Solid Edge part; units mm, degrees
sketch "Sketch1" plane through (0, 0, 0) normal (0, -1, 0) x (1, 0, 0)
  line L0 (30, 0) -> (18.9422, 160.02)
  line L1 (-19.0139, 161.311) -> (-20, 0)
  line L2 (30, 0) -> (-20, 0)
  arc A0 (-19.0139, 161.311) -> (18.9422, 160.02) centre (-0.0578, 160.02) cw
extrude "Protrusion1" add sketch "Sketch1" against normal blind 10
sketch "Sketch2" plane through (0, 0, 0) normal (0, -1, 0) x (1, 0, 0)
  circle A0 centre (0, 160) radius 10
extrude "ExtrudedCutout_1" cut sketch "Sketch2" against normal blind 10
hole "Hole_1" at (-15.5, 0, 5.5) direction (0, 1, 0) diameter 3.2 end through all counterbore diameter 5.8 counterbore depth 3.4
pattern_linear "Pattern1" count 2 spacing 31 along (1, 0, 0) count 2 spacing 31 along (0, 0, 1) of "Hole_1"
hole "Hole_2" at (0, 10, 21) direction (0, -1, 0) diameter 5.5 end through all counterbore diameter 23 counterbore depth 3
sketch "Sketch3" plane through (0, 0, 89.51) normal (0, -1, 0) x (1, 0, 0)
  line L0 (9.2202, -0.4765) -> (6.2316, -0.7379)
  line L1 (6.1009, 0.7564) -> (6.2316, -0.7379)
  line L2 (14.0705, 1.4536) -> (6.1009, 0.7564)
  line L3 (14.2012, -0.0407) -> (14.0705, 1.4536)
  line L4 (9.2202, -0.4765) -> (14.2012, -0.0407)
  line L5 (14.7241, -6.0178) -> (9.7432, -6.4536)
  line L6 (9.7432, -6.4536) -> (9.3074, -1.4727)
  line L7 (14.2883, -1.0369) -> (9.3074, -1.4727)
  line L8 (14.7241, -6.0178) -> (14.2883, -1.0369)
  line L9 (9.8303, -7.4498) -> (14.8113, -7.014)
  line L10 (14.942, -8.5083) -> (14.8113, -7.014)
  line L11 (6.9725, -9.2056) -> (14.942, -8.5083)
  line L12 (6.8417, -7.7113) -> (6.9725, -9.2056)
  line L13 (6.8417, -7.7113) -> (9.8303, -7.4498)
extrude "ExtrudedProtrusion_2" add sketch "Sketch3" along normal blind 8
sketch "Sketch4" plane through (0, 0, 89.51) normal (0, -1, 0) x (1, 0, 0)
  circle A0 centre (15.8473, -0.0407) radius 1
  circle A1 centre (16.3289, -6.7414) radius 1
extrude "ExtrudedCutout_3" cut sketch "Sketch4" against normal blind 10
sketch "Sketch5" plane through (12.0158, -8, 85.7648) normal (0, -1, 0) x (0.9962, 0, 0.0872)
  line L0 (-5.5, 5) -> (-5.5, -5)
  line L1 (-5.5, -5) -> (2.5, -5)
  line L2 (2.5, -5) -> (2.5, 5)
  line L3 (2.5, 5) -> (-5.5, 5)
extrude "ExtrudedProtrusion_3" add sketch "Sketch5" along normal blind 3
sketch "Sketch6" plane through (0, 0, 89.51) normal (0, -1, 0) x (1, 0, 0)
  line L0 (-12.7631, 16.3965) -> (-4.7936, 15.6993)
  line L1 (-4.7936, 15.6993) -> (-4.9243, 14.205)
  line L2 (-4.9243, 14.205) -> (-12.8939, 14.9022)
  line L3 (-12.8939, 14.9022) -> (-12.7631, 16.3965)
  line L4 (-8.4358, 8.4893) -> (-8, 13.4703)
  line L5 (-8, 13.4703) -> (-12.981, 13.906)
  line L6 (-12.981, 13.906) -> (-13.4168, 8.9251)
  line L7 (-13.4168, 8.9251) -> (-8.4358, 8.4893)
  line L8 (-13.5039, 7.9289) -> (-5.5344, 7.2316)
  line L9 (-5.5344, 7.2316) -> (-5.6651, 5.7373)
  line L10 (-5.6651, 5.7373) -> (-13.6347, 6.4346)
  line L11 (-13.6347, 6.4346) -> (-13.5039, 7.9289)
extrude "ExtrudedProtrusion_4" add sketch "Sketch6" along normal blind 8
sketch "Sketch7" plane through (-10.7084, -8, 100.7077) normal (0, -1, 0) x (0.9962, 0, -0.0872)
  line L0 (5.5, 5) -> (5.5, -5)
  line L1 (5.5, -5) -> (-2.5, -5)
  line L2 (-2.5, -5) -> (-2.5, 5)
  line L3 (-2.5, 5) -> (5.5, 5)
extrude "ExtrudedProtrusion_5" add sketch "Sketch7" along normal blind 3
hole "Hole1" at (-14.1769, 0, 104.0133) direction (0, 1, 0) diameter 2 end up to next
hole "Hole2" at (-14.7852, 0, 97.9993) direction (0, 1, 0) diameter 2 end up to next
fillet "Round_1" [suppressed]
fillet "Round_2" radius 1 4 edges at (-8.7783, -11, 105.5579) (-13.1989, -11, 100.9256) (-9.6499, -11, 95.596) (-5.2293, -11, 100.2283)
fillet "Round_3" radius 1 4 edges at (10.0857, -11, 90.615) (6.5367, -11, 85.2854) (10.9572, -11, 80.653) (14.5062, -11, 85.9826)
fillet "Round_4" [suppressed]
Part model, mm, in its own coordinate system. A direction names the side the tool comes from. Coordinates: 2 decimals unless noted, no trailing zeros. Loops run counter-clockwise (first coordinate to the right, second up) from the corner with the lowest first, then second, coordinate; pieces in that order, holes last. Notation, with made-up numbers: M 30,37 L 80,37 A18 cw 80,67 Z; hole C 19.5,81.5 d5. An arc over 180 degrees is marked long. Use a Markdown table: item, result. Add a question column.
Q1. Cut at A-A (z = 36.5). Write the cut outline in (x, y).
Q2. Probe L1, parallel to Z at x = 0, y = 4; L2, parallel to Z at x = 0, y = 8; L3, parallel to Z at x = -15.5, y = 1.1. List the from-to ranges inside material, lowest first.
Q3. Which spindle directions (+Z, -Z, +X, -X, +Y, -Y) get a long thin tool onto all of the face, cutting with end or side? Do faces 1 (the flat face through (-14, 3.4, 4)), 2 (the flat face through (-9.59, -3.94, 95.59)), 3 (the flat face through (10.9, -3.94, 80.65)). Say none if no direction does.
Q4. Cut at D-D (z = 58.5). Write the cut outline in (x, y).
Q5. Pin check, flat tips, straight feed: P1, Ø2, axis at x = 6.5, z = 75, coming from the -Y side; P2, Ø7, axis at x = 0, z = 21, coming from the +Y side; P3, Ø6, axis at x = 12, y = -2, coming from the +Z side; P4, Ø1.8, axis at x = 15.85, z = 89.47, coming from the +Y side. Stop position of each tip, or through.
Q6. Cut at B-B (x = 0). Write the cut outline in (y, z).
Q7. Mould opens along Y. For faces 4 (the flat face through (2.4, 7, 23.4)), 5 (the flat face through (-8.22, -3.94, 100.45)), 6 (the flat face through (11, -11, 86)), 7 (the flat face through (10.14, -3.94, 90.62)) say: +Y half, -Y half, draft (parallel to the pull), parting line (faces both ways), or undercut.
Q8. Cut at C-C (z = 165.5). Write the cut outline in (x, y), and give its area (3 significant figures).
Worked out:
| question | item | result |
|---|---|---|
| 1 | outline | M -19.78,0 L -18.4,0 L -18.4,3.4 L -17.1,3.4 L -17.1,10 L -19.78,10 Z; M -13.9,3.4 L -12.6,3.4 L -12.6,0 L 12.6,0 L 12.6,3.4 L 13.9,3.4 L 13.9,10 L -13.9,10 Z; M 17.1,3.4 L 18.4,3.4 L 18.4,0 L 27.48,0 L 27.48,10 L 17.1,10 Z |
| 2 | L1 | z = 0 to 18.25, 23.75 to 150, 170 to 179.02 |
| 2 | L2 | z = 0 to 9.5, 32.5 to 150, 170 to 179.02 |
| 2 | L3 | z = 0 to 2.6, 8.4 to 33.6, 39.4 to 97.3, 98.7 to 171.09 |
| 3 | face 1 | -Y |
| 3 | face 2 | -Z, -X, -Y |
| 3 | face 3 | -Z, +X, -Y |
| 4 | outline | M -19.64,0 L 25.96,0 L 25.96,10 L -19.64,10 Z |
| 5 | P1 | stops at y = 0 |
| 5 | P2 | stops at y = 7 |
| 5 | P3 | stops at z = 176.28 |
| 5 | P4 | passes through |
| 6 | outline | M 0,0 L 10,0 L 10,9.5 L 7,9.5 L 7,18.25 L 0,18.25 Z; M 0,23.75 L 7,23.75 L 7,32.5 L 10,32.5 L 10,150 L 0,150 Z; M 0,170 L 10,170 L 10,179.02 L 0,179.02 Z |
| 7 | face 4 | +Y half |
| 7 | face 5 | undercut |
| 7 | face 6 | -Y half |
| 7 | face 7 | draft |
| 8 | outline | M -18.25,0 L -8.35,0 L -8.35,10 L -18.25,10 Z; M 8.35,0 L 18.13,0 L 18.13,10 L 8.35,10 Z |
| 8 | area | 197 mm2 |
